Geometry check sheet. Reference: the model listing, model coordinates, mm. A direction names the side the tool comes from. Round coordinates to 2 decimals unless told otherwise and drop trailing zeros. Order: outer loops, then holes, each group sorted by start corner. A loop starts at its lowest first (then second) coordinate and runs counter-clockwise, first axis right, second up. Notation, with made-up numbers: (-2, 57) - (32, 57) arc R11 cw to (32, 63) - close; hole circle Ø10 at (62.5, 80.25). An arc over 180 degrees is marked (long way). Write each question's results on one line, items separated by ' | '.
```python
from build123d import *

# Parameters (mm, degrees)
CUT_EXTRUDE1_DEPTH      = 84.815273071
CUT_EXTRUDE1_DEPTH_BACK = 84.815273071
SKETCH3_R               = 30


with BuildPart() as part:
    # Sketch1 → Revolve1 (revolve)
    with BuildSketch(Plane.XY, mode=Mode.PRIVATE) as revolve1_sk:
        with BuildLine():
            Line((0, 45), (-50, 45))
            Line((-50, 45), (-50, 40))
            Line((-50, 40), (-35, 40))
            Line((-35, 40), (-35, 35))
            Line((-35, 35), (-33, 35))
            Line((-33, 35), (-33, 25))
            Line((-33, 25), (-45.073826017, 5.207769821))
            ThreePointArc((-45.073826017, 5.207769821), (-46.536898379, 0), (-45.073826017, -5.207769821))
            Line((-45.073826017, -5.207769821), (-33, -25))
            Line((-33, -25), (-33, -40))
            Line((-33, -40), (0, -40))
            Line((0, -40), (0, 45))
        make_face()
    revolve(revolve1_sk.sketch.rotate(Axis((0, 78.93258427, 0), (0, -1, 0)), 270), axis=Axis((0, 78.93258427, 0), (0, -1, 0)))

    # Sketch3 → Cut-Extrude1 (cut, two sides: drawn at the far end of the back side and taken through both)
    with BuildSketch(Plane(origin=(0, 0, 0), x_dir=(1, 0, 0), z_dir=(0, 1, 0)).offset(-CUT_EXTRUDE1_DEPTH_BACK)):
        with Locations(Location((0, 0, 0), (0, 0, 270))):
            Circle(SKETCH3_R)
    extrude(amount=CUT_EXTRUDE1_DEPTH + CUT_EXTRUDE1_DEPTH_BACK, mode=Mode.SUBTRACT)


solid = part.part
```
(1) Depth check by flat-ended pin: pin 1 Ø8 at (x, y) = (-27.5, -8.5) entering from +Z; pin 2 Ø6 at (x, y) = (33, 2.5) entering from +Z; pin 3 Ø10 at (x, y) = (7, -29) entering from -Z. Enter the tip coordinate at first touch or a pass-through.
Answers follow:
pin 1: z = 37.39 | pin 2: z = 35.29 | pin 3: z = -33.02
(2) Draft check along Z on faces 4 (the face through (1.32, 1.9, -29.97)), 5 (the face through (27, -40, 15)), 6 (the face through (32.215, 29.93, -7.154)). Enter one of: released by +Z, released by -Z, zero draft, split by the parting line, or undercut.
Answers follow:
face 4: undercut | face 5: zero draft | face 6: split by the parting line
(3) Section check B-B (z = 0). Record the cut outline in (x, y).
Answers follow:
outline: (-50, 40) - (-35, 40) - (-35, 35) - (-33, 35) - (-33, 25) - (-45.07, 5.21) arc R10 ccw to (-45.07, -5.21) - (-33, -25) - (-33, -40) - (-30, -40) - (-30, 45) - (-50, 45) - close; (30, -40) - (33, -40) - (33, -25) - (45.07, -5.21) arc R10 ccw to (45.07, 5.21) - (33, 25) - (33, 35) - (35, 35) - (35, 40) - (50, 40) - (50, 45) - (30, 45) - close
(4) Access from +Z, -Z, +X, -X, +Y, -Y to the whole of each face (thin tool, end or side, straight path). Record for faces 1 (the face through (32.215, -32.605, -7.154)), 2 (the face through (21, 37, -28)), 3 (the face through (-15.02, 42.46, 47.69)).
Answers follow:
face 1: -Y | face 2: none | face 3: +Y, -Y
(5) Section check A-A (x = 0). Record the cut outline in (y, z).
Answers follow:
outline: (-40, -33) - (-25, -33) - (-5.21, -45.07) arc R10 ccw to (5.21, -45.07) - (25, -33) - (35, -33) - (35, -35) - (40, -35) - (40, -50) - (45, -50) - (45, -30) - (-40, -30) - close; (-40, 30) - (45, 30) - (45, 50) - (40, 50) - (40, 35) - (35, 35) - (35, 33) - (25, 33) - (5.21, 45.07) arc R10 ccw to (-5.21, 45.07) - (-25, 33) - (-40, 33) - close
(6) Section check D-D (y = -15). Record the cut outline in (x, z), then the cut area to 3 significant figures.
Answers follow:
outline: circle Ø78.2 at (0, 0); hole circle Ø60 at (0, 0) | area: 1,980 mm²
(7) Section check C-C (y = 3.5). Record the cut outline in (x, z).
Answers follow:
outline: circle Ø91.81 at (0, 0); hole circle Ø60 at (0, 0)
(8) Material ranges on line 1 (Y direction, x = 26.5, z = -21.5); line 2 (Y direction, x = -40.5, z = 4); line 3 (X direction, y = 24, z = 0), recorded low to high.
Answers follow:
line 1: -23.16 to 23.16, 35 to 45 | line 2: -12.38 to 12.38, 40 to 45 | line 3: -33.61 to -30, 30 to 33.61
